The figure shows three views and two pictorial views of one solid part (mm, origin at its lowest corner). Answer the questions. A direction names the side the tool comes from. Give positions to 0.01 mm unless a question says otherwise; leave off trailing zeros. Loops run counter-clockwise (first coordinate to the right, second up) from the corner with the lowest first, then second, coordinate; pieces in that order, holes last. Notation, with made-up numbers: (64, 24.25) - (88, 24.25) arc R18 ccw to (88, 39.25) - close; hole circle Ø1 at (-23, -19). An arc over 180 degrees is marked (long way). Write item = value, one per line.
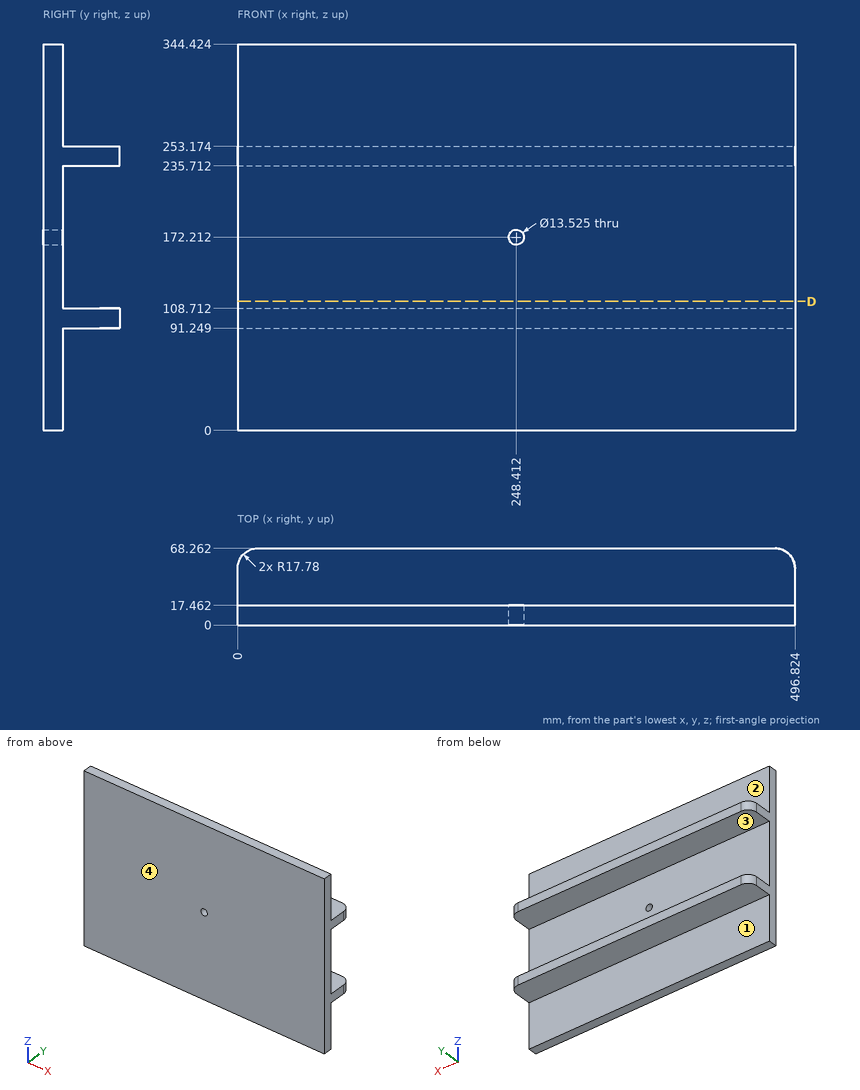
1) A cutting plane is placed at D-D on z = 115. Determine the outline of the cut face in (x, y) (1 decimal).
Output:
outline = (0, 0) - (496.8, 0) - (496.8, 17.5) - (0, 17.5) - close
2) Find the intervals of material crossed by probe 1 along Y at (x, z) = (306.5, 136.5), in increasing order.
Output:
probe_1 = 0 to 17.46
3) A tool of negligible diameter and unlimited length cuts with its end or side. For the marked faces 1, 2, 3 and 4, from which of +Z, -Z, +X, -X, +Y, -Y can it reach the whole face along a straight path? Write none if from no direction.
Output:
face_1 = -Z, +X, -X, +Y
face_2 = +Z, +X, -X, +Y
face_3 = +X, -X, +Y
face_4 = +Z, -Z, +X, -X, -Y
4) This flat-tipped pin is pushed along its axis until it touches: P1, Ø12, axis at x = 108.5, z = 131.5, coming from the +Y side. Where does it stop, or does it pass through?
Output:
P1 = 17.46
